The model under review builds one solid part; all positions refer to its coordinate system, in mm. Face numbers are marked on the shaded views. A direction names the side the tool comes from. Coordinates: 2 decimals unless noted, no trailing zeros. Write each loop counter-clockwise with the first axis right and the second up, starting at its lowest first coordinate (ties: lowest second). Pieces come first, ordered by that corner, then holes.
1) For P1, Ø8, axis at x = -7, y = -11.5, coming from the +Z side; P2, Ø15, axis at x = -3, y = 1, coming from the +Z side, all flat-tipped, find the tip position at first contact; note any pin that passes through.
2) Machinability: for the marked faces 4 and 5, which of the approach directions +Z, -Z, +X, -X, +Y, -Y give a long, thin tool a straight path to every point of the face, cutting with its end or side? Answer none if there is none.
3) For line 1 (Y direction, x = 0, z = -1.5); line 2 (X direction, y = 0, z = -4.25) (3 decimals); line 3 (Y direction, x = -4, z = 15.5), list the stretches that pass through material, from the lowest coordinate up.
4) Mouldability with a two-part tool opening along Y and no side actions: class the marked faces 1, 2 and 3 as released by +Y, released by -Y, zero draft, split by the parting line, or undercut.
5) Add section A-A, the plane z = 5.5. State the section outline as (x, y) points (3 decimals), then the cut area to 3 significant figures.
6) Add section C-C, the plane z = -2.25. State the section outline as (x, y) points (3 decimals), then the cut area to 3 significant figures.
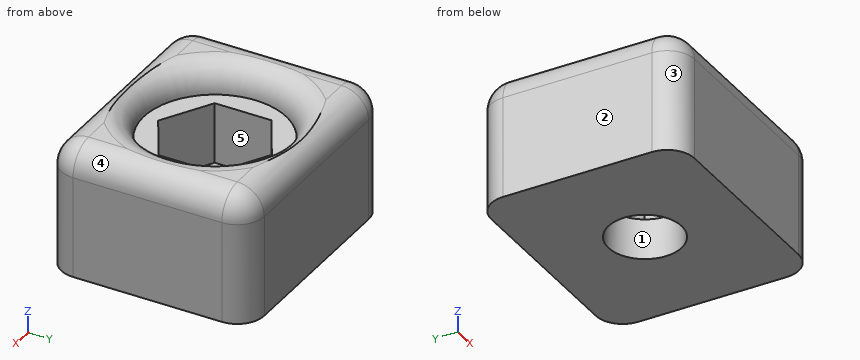
from build123d import *

# Parameters (mm, degrees)
F0_W         = 44.45
F0_H         = 38.1
F1_DEPTH     = 16.51
F3_DEPTH     = 25.4
F4_R         = 13.335
F5_DEPTH     = 5.08
F6_F1_R      = 5.0799
F6_T2_DEPTH  = 69.85
F6_T4_DEPTH  = 69.85
F6_T6_DEPTH  = 27.94
F6_T8_DEPTH  = 24.13
F6_T11_ANGLE = 90
F6_T13_ANGLE = 90
F6_T14_DEPTH = 27.94
F6_T16_DEPTH = 24.13
F6_T19_ANGLE = 90
F6_T21_ANGLE = 90
F8_R         = 6.858
F9_DEPTH     = 7.62


# Not quite as in the source:
# - a fillet or chamfer that OpenCascade refuses, or shapes differently, is made with other operations: its cross-section is extruded or revolved along the edge and cut away or added
# - a fillet or chamfer is up to 0.001 mm smaller than in the source, because OpenCascade refuses the exact size
# - a feature of the source that left no trace in its solid (it failed there, or was rolled back) is left out


with BuildPart() as f1:
    # F0 (on Top) → F1 (new body)
    with BuildSketch(Plane.XY):
        Rectangle(F0_W, F0_H)
    extrude(amount=F1_DEPTH)

    # F2 (on face) → F3 (cut)
    with BuildSketch(Plane.XY.offset(16.51)):
        Polygon((9.2387590076, 5.334), (0, 10.668), (-9.2387590076, 5.334), (-9.2387590076, -5.334), (0, -10.668), (9.2387590076, -5.334), align=None)
    extrude(amount=-F3_DEPTH, mode=Mode.SUBTRACT)

    # F4 (on face) → F5 (cut)
    with BuildSketch(Plane.XY.offset(16.51)):
        Circle(F4_R)
        Polygon((-9.2387590076, 5.334), (0, 10.668), (9.2387590076, 5.334), (9.2387590076, -5.334), (0, -10.668), (-9.2387590076, -5.334), align=None, mode=Mode.SUBTRACT)
    extrude(amount=-F5_DEPTH, mode=Mode.SUBTRACT)

    # F6: fillet of radius 5.08 on 5 edges, made by hand

    # F6_f1 (radius 5.08 in the source; OpenCascade refuses exactly that, so slightly less here)
    f6_f1_edges = [f1.edges().sort_by_distance(p)[0] for p in [
        (-13.335, 0, 16.51),
    ]]
    fillet(f6_f1_edges, radius=F6_F1_R)

    # F6_s3 → F6_t2 (cut)
    with BuildSketch(Plane.YZ.offset(-34.925)):
        with BuildLine():
            ThreePointArc((13.97, 16.51), (17.5621024484, 15.0221024484), (19.05, 11.43))
            Line((19.05, 11.43), (19.1516, 11.43))
            Line((19.1516, 11.43), (19.1516, 16.6116))
            Line((19.1516, 16.6116), (13.97, 16.6116))
            Line((13.97, 16.6116), (13.97, 16.51))
        make_face()
    extrude(amount=F6_T2_DEPTH, mode=Mode.SUBTRACT)

    # F6_s5 → F6_t4 (cut)
    with BuildSketch(Plane.YZ.offset(-34.925)):
        with BuildLine():
            ThreePointArc((-13.97, 16.51), (-17.5621024484, 15.0221024484), (-19.05, 11.43))
            Line((-19.05, 11.43), (-19.1516, 11.43))
            Line((-19.1516, 11.43), (-19.1516, 16.6116))
            Line((-19.1516, 16.6116), (-13.97, 16.6116))
            Line((-13.97, 16.6116), (-13.97, 16.51))
        make_face()
    extrude(amount=F6_T4_DEPTH, mode=Mode.SUBTRACT)

    # F6_s7 → F6_t6 (cut)
    with BuildSketch(Plane.XZ.offset(-13.97)):
        with BuildLine():
            ThreePointArc((17.145, 16.51), (20.7371024484, 15.0221024484), (22.225, 11.43))
            Line((22.225, 11.43), (22.3266, 11.43))
            Line((22.3266, 11.43), (22.3266, 16.6116))
            Line((22.3266, 16.6116), (17.145, 16.6116))
            Line((17.145, 16.6116), (17.145, 16.51))
        make_face()
    extrude(amount=F6_T6_DEPTH, mode=Mode.SUBTRACT)

    # F6_s9 → F6_t8 (cut)
    with BuildSketch(Plane.XY.offset(-12.7)):
        with BuildLine():
            ThreePointArc((22.225, 13.97), (20.7371024484, 17.5621024484), (17.145, 19.05))
            Line((17.145, 19.05), (17.145, 19.1516))
            Line((17.145, 19.1516), (22.3266, 19.1516))
            Line((22.3266, 19.1516), (22.3266, 13.97))
            Line((22.3266, 13.97), (22.225, 13.97))
        make_face()
        with BuildLine():
            ThreePointArc((22.225, -13.97), (20.7371024484, -17.5621024484), (17.145, -19.05))
            Line((17.145, -19.05), (17.145, -19.1516))
            Line((17.145, -19.1516), (22.3266, -19.1516))
            Line((22.3266, -19.1516), (22.3266, -13.97))
            Line((22.3266, -13.97), (22.225, -13.97))
        make_face()
    extrude(amount=F6_T8_DEPTH, mode=Mode.SUBTRACT)

    # F6_s10 → F6_t11 (revolve, cut)
    with BuildSketch(Plane.XY.offset(11.43)):
        with BuildLine():
            ThreePointArc((22.225, -13.97), (20.7371024484, -17.5621024484), (17.145, -19.05))
            Line((17.145, -19.05), (17.145, -19.1516))
            Line((17.145, -19.1516), (22.3266, -19.1516))
            Line((22.3266, -19.1516), (22.3266, -13.97))
            Line((22.3266, -13.97), (22.225, -13.97))
        make_face()
    revolve(axis=Axis((22.225, -13.97, 11.43), (-1, 0, 0)), revolution_arc=F6_T11_ANGLE, mode=Mode.SUBTRACT)

    # F6_s12 → F6_t13 (revolve, cut)
    with BuildSketch(Plane.XY.offset(11.43)):
        with BuildLine():
            ThreePointArc((17.145, 19.05), (20.7371024484, 17.5621024484), (22.225, 13.97))
            Line((22.225, 13.97), (22.3266, 13.97))
            Line((22.3266, 13.97), (22.3266, 19.1516))
            Line((22.3266, 19.1516), (17.145, 19.1516))
            Line((17.145, 19.1516), (17.145, 19.05))
        make_face()
    revolve(axis=Axis((22.225, 13.97, 11.43), (1, 0, 0)), revolution_arc=F6_T13_ANGLE, mode=Mode.SUBTRACT)

    # F6_s15 → F6_t14 (cut)
    with BuildSketch(Plane.XZ.offset(-13.97)):
        with BuildLine():
            ThreePointArc((-17.145, 16.51), (-20.7371024484, 15.0221024484), (-22.225, 11.43))
            Line((-22.225, 11.43), (-22.3266, 11.43))
            Line((-22.3266, 11.43), (-22.3266, 16.6116))
            Line((-22.3266, 16.6116), (-17.145, 16.6116))
            Line((-17.145, 16.6116), (-17.145, 16.51))
        make_face()
    extrude(amount=F6_T14_DEPTH, mode=Mode.SUBTRACT)

    # F6_s17 → F6_t16 (cut)
    with BuildSketch(Plane.XY.offset(-12.7)):
        with BuildLine():
            ThreePointArc((-22.225, -13.97), (-20.7371024484, -17.5621024484), (-17.145, -19.05))
            Line((-17.145, -19.05), (-17.145, -19.1516))
            Line((-17.145, -19.1516), (-22.3266, -19.1516))
            Line((-22.3266, -19.1516), (-22.3266, -13.97))
            Line((-22.3266, -13.97), (-22.225, -13.97))
        make_face()
        with BuildLine():
            ThreePointArc((-17.145, 19.05), (-20.7371024484, 17.5621024484), (-22.225, 13.97))
            Line((-22.225, 13.97), (-22.3266, 13.97))
            Line((-22.3266, 13.97), (-22.3266, 19.1516))
            Line((-22.3266, 19.1516), (-17.145, 19.1516))
            Line((-17.145, 19.1516), (-17.145, 19.05))
        make_face()
    extrude(amount=F6_T16_DEPTH, mode=Mode.SUBTRACT)

    # F6_s18 → F6_t19 (revolve, cut)
    with BuildSketch(Plane.XY.offset(11.43)):
        with BuildLine():
            ThreePointArc((-17.145, 19.05), (-20.7371024484, 17.5621024484), (-22.225, 13.97))
            Line((-22.225, 13.97), (-22.3266, 13.97))
            Line((-22.3266, 13.97), (-22.3266, 19.1516))
            Line((-22.3266, 19.1516), (-17.145, 19.1516))
            Line((-17.145, 19.1516), (-17.145, 19.05))
        make_face()
    revolve(axis=Axis((-22.225, 13.97, 11.43), (1, 0, 0)), revolution_arc=F6_T19_ANGLE, mode=Mode.SUBTRACT)

    # F6_s20 → F6_t21 (revolve, cut)
    with BuildSketch(Plane.XY.offset(11.43)):
        with BuildLine():
            ThreePointArc((-17.145, -19.05), (-20.7371024484, -17.5621024484), (-22.225, -13.97))
            Line((-22.225, -13.97), (-22.3266, -13.97))
            Line((-22.3266, -13.97), (-22.3266, -19.1516))
            Line((-22.3266, -19.1516), (-17.145, -19.1516))
            Line((-17.145, -19.1516), (-17.145, -19.05))
        make_face()
    revolve(axis=Axis((-22.225, -13.97, 11.43), (-1, 0, 0)), revolution_arc=F6_T21_ANGLE, mode=Mode.SUBTRACT)

    # F8 (on face) → F9 (join)
    with BuildSketch(Plane(origin=(0, 0, 0), x_dir=(1, 0, 0), z_dir=(0, 0, -1))):
        with BuildLine():
            Line((-17.145, -19.05), (17.145, -19.05))
            ThreePointArc((17.145, -19.05), (20.7371024484, -17.5621024484), (22.225, -13.97))
            Line((22.225, -13.97), (22.225, 13.97))
            ThreePointArc((22.225, 13.97), (20.7371024484, 17.5621024484), (17.145, 19.05))
            Line((17.145, 19.05), (-17.145, 19.05))
            ThreePointArc((-17.145, 19.05), (-20.7371024484, 17.5621024484), (-22.225, 13.97))
            Line((-22.225, 13.97), (-22.225, -13.97))
            ThreePointArc((-22.225, -13.97), (-20.7371024484, -17.5621024484), (-17.145, -19.05))
        make_face()
        Polygon((9.2387590076, 5.334), (9.2387590076, -5.334), (0, -10.668), (-9.2387590076, -5.334), (-9.2387590076, 5.334), (0, 10.668), align=None, mode=Mode.SUBTRACT)
        Polygon((0, -10.668), (9.2387590076, -5.334), (9.2387590076, 5.334), (0, 10.668), (-9.2387590076, 5.334), (-9.2387590076, -5.334), align=None)
        Circle(F8_R, mode=Mode.SUBTRACT)
    extrude(amount=F9_DEPTH)


solid = f1.part
Geometry results:
1. P1: stops at z = 16.42
1. P2: stops at z = 11.43
2. face 4: +Z, +X, +Y, -Y
2. face 5: +Z
3. line 1: y = -19.05 to -6.86, 6.86 to 19.05
3. line 2: x = -22.225 to -6.858, 6.858 to 22.225
3. line 3: y = -17.01 to -14.85, 14.85 to 17.01
4. face 1: undercut
4. face 2: zero draft
4. face 3: released by -Y
5. outline: (-22.225, -13.97) arc R5.08 ccw to (-17.145, -19.05) - (17.145, -19.05) arc R5.08 ccw to (22.225, -13.97) - (22.225, 13.97) arc R5.08 ccw to (17.145, 19.05) - (-17.145, 19.05) arc R5.08 ccw to (-22.225, 13.97) - close; hole (-9.239, -5.334) - (0, -10.668) - (9.239, -5.334) - (9.239, 5.334) - (0, 10.668) - (-9.239, 5.334) - close
5. area: 1,380 mm2
6. outline: (-22.225, -13.97) arc R5.08 ccw to (-17.145, -19.05) - (17.145, -19.05) arc R5.08 ccw to (22.225, -13.97) - (22.225, 13.97) arc R5.08 ccw to (17.145, 19.05) - (-17.145, 19.05) arc R5.08 ccw to (-22.225, 13.97) - close; hole circle Ø13.716 at (0, 0)
6. area: 1,520 mm2
